Geometry check sheet. Reference: the model listing, model coordinates, mm. A direction names the side the tool comes from. Coordinates: 2 decimals unless noted, no trailing zeros. Return JSON: item names as keys, results as strings. Group by question number.
Item 1: Draft check along X on faces 1 (the flat face through (13, 0, 188)), 2 (the flat face through (3.175, 13, 188)), 3 (the flat face through (0, 13, 188)). Enter one of: pulls with the +X half, pulls with the -X half, needs draft (parallel to the pull), parting line crosses it, or undercut.
Item 2: Tool access check on faces 4 (the flat face through (22.225, 13, 188)), 5 (the flat face through (25.4, 13, 188)). Record the directions out of +Z, -Z, +X, -X, +Y, -Y that give a thin tool (end or side, any length) a straight path to the whole face; none if there is none.
Item 3: Scan lines: probe 1 along X at (y, z) = (21, 205.5) (3 decimals); probe 2 along Y at (x, z) = (1.4, 152.4). Record each from-to range of solid material in increasing order.
Autodesk Inventor part; units mm, degrees
ref_plane "YZ Plane" through (0, 0, 0) normal (1, 0, 0) x (0, 1, 0)
ref_plane "XZ Plane" through (0, 0, 0) normal (0, 1, 0) x (-1, 0, 0)
ref_plane "XY Plane" through (0, 0, 0) normal (0, 0, 1) x (1, 0, 0)
sketch "Sketch1" plane through (0, 0, 0) normal (0, 0, 1) x (1, 0, 0)
  line L0 (0, 0) -> (25.4, 0)
  line L1 (25.4, 0) -> (25.4, 25.4)
  line L2 (25.4, 25.4) -> (0, 25.4)
  line L3 (0, 25.4) -> (0, 0)
  line L4 (3.175, 22.225) -> (22.225, 22.225)
  line L5 (22.225, 22.225) -> (22.225, 3.175)
  line L6 (22.225, 3.175) -> (3.175, 3.175)
  line L7 (3.175, 3.175) -> (3.175, 22.225)
  dimension "d0" = 25.4
  dimension "d1" = 25.4
  dimension "d2" = 3.175
extrude "Extrusion1" add sketch "Sketch1" along normal blind 381
sketch "Sketch2" plane through (25.4, 0, 0) normal (1, 0, 0) x (0, 0, -1)
  line L0 (0, 0) -> (0, 25.4)
  line L1 (-381, 0) -> (-381, 25.4)
  line L2 (0, 0) -> (-381, 0)
  circle A0 centre (-368.3, 12.7) radius 2.0701
  circle A1 centre (-355.6, 12.7) radius 2.0701
  circle A2 centre (-342.9, 12.7) radius 2.0701
  circle A3 centre (-330.2, 12.7) radius 2.0701
  circle A4 centre (-317.5, 12.7) radius 2.0701
  circle A5 centre (-304.8, 12.7) radius 2.0701
  circle A6 centre (-292.1, 12.7) radius 2.0701
  circle A7 centre (-279.4, 12.7) radius 2.0701
  circle A8 centre (-266.7, 12.7) radius 2.0701
  circle A9 centre (-190.5, 12.7) radius 2.0701
  circle A10 centre (-177.8, 12.7) radius 2.0701
  circle A11 centre (-165.1, 12.7) radius 2.0701
  circle A12 centre (-152.4, 12.7) radius 2.0701
  circle A13 centre (-139.7, 12.7) radius 2.0701
  circle A14 centre (-12.7, 12.7) radius 2.0701
  circle A15 centre (-38.1, 12.7) radius 2.0701
  dimension "d5" = 4.1402
  dimension "d6" = 12.7
  dimension "d7" = 12.7
  dimension "d10" = 12.7
  dimension "d15" = 76.2
  dimension "d16" = 12.7
  dimension "d19" = 12.7
  dimension "d24" = 12.7
  dimension "d25" = 12.7
  dimension "d28" = 25.4
extrude "Extrusion2" cut sketch "Sketch2" against normal blind 381
sketch "Sketch3" plane through (0, 25.4, 0) normal (0, 1, 0) x (1, 0, 0)
  line L0 (25.4, 0) -> (0, 0)
  line L1 (25.4, -381) -> (0, -381)
  line L2 (25.4, 0) -> (25.4, -381)
  circle A0 centre (12.7, -304.8) radius 2.0701
  circle A1 centre (12.7, -292.1) radius 2.0701
  circle A2 centre (12.7, -279.4) radius 2.0701
  circle A3 centre (12.7, -266.7) radius 2.0701
  circle A4 centre (12.7, -254) radius 2.0701
  circle A5 centre (12.7, -241.3) radius 2.0701
  circle A6 centre (12.7, -50.8) radius 2.0701
  circle A7 centre (12.7, -63.5) radius 2.0701
  circle A8 centre (12.7, -76.2) radius 2.0701
  circle A9 centre (12.7, -88.9) radius 2.0701
  circle A10 centre (12.7, -101.6) radius 2.0701
  circle A11 centre (12.7, -114.3) radius 2.0701
  circle A12 centre (12.7, -127) radius 2.0701
  circle A13 centre (12.7, -165.1) radius 2.0701
  dimension "d35" = 4.1402
  dimension "d36" = 76.2
  dimension "d37" = 12.7
  dimension "d40" = 12.7
  dimension "d45" = 50.8
  dimension "d46" = 12.7
  dimension "d49" = 12.7
  dimension "d54" = 38.1
  dimension "d55" = 12.7
extrude "Extrusion3" cut sketch "Sketch3" against normal blind 381
properties part number "Vertical 15 in Segments (2)"
Computed:
{
 "1": {"face 1": "needs draft", "face 2": "undercut", "face 3": "pulls with the -X half"},
 "2": {"face 4": "+Z, -Z", "face 5": "+Z, -Z, +X, +Y, -Y"},
 "3": {"probe 1": "x = 0 to 3.175, 22.225 to 25.4", "probe 2": "y = 0 to 10.63, 14.77 to 25.4"}
}
